Read the model definition and answer for the solid it produces. Units are mm, in the model's axes. A direction names the side the tool comes from. Give positions to 0.01 mm unless a question says otherwise; leave off trailing zeros. Order: outer loops, then holes, each group sorted by start corner. A loop starts at its lowest first (then second) coordinate and runs counter-clockwise, first axis right, second up. Notation, with made-up numbers: M 71.25,-34 L 104.25,-34 A17 cw 104.25,-5 Z; hole C 86.5,-12.75 d4. An arc over 180 degrees is marked long. One line per item, written item: value.
Solid Edge part; units mm, degrees
sketch "Sketch1" plane through (0, 0, 0) normal (0, 0, 1) x (1, 0, 0)
  circle A0 centre (0, 0) radius 62.5
  circle A1 centre (-39.7748, -39.7748) radius 1.5
  circle A2 centre (39.7748, -39.7748) radius 1.5
  circle A3 centre (39.7748, 39.7748) radius 1.5
  circle A4 centre (-39.7748, 39.7748) radius 1.5
extrude "Protrusion1" add sketch "Sketch1" along normal blind 75
sketch "Sketch2" plane through (0, 0, 75) normal (0, 0, 1) x (1, 0, 0)
  arc A0 (-37.0362, 42.3365) -> (37.0362, 42.3365) centre (0, 0) cw
  arc A1 (42.3365, 37.0362) -> (42.3365, -37.0362) centre (0, 0) cw
  arc A2 (37.0362, -42.3365) -> (-37.0362, -42.3365) centre (0, 0) cw
  arc A3 (-42.3365, -37.0362) -> (-42.3365, 37.0362) centre (0, 0) cw
  arc A4 (-37.0362, 42.3365) -> (-42.3365, 37.0362) centre (-39.7748, 39.7748) cw
  arc A5 (42.3365, 37.0362) -> (37.0362, 42.3365) centre (39.7748, 39.7748) cw
  arc A6 (37.0362, -42.3365) -> (42.3365, -37.0362) centre (39.7748, -39.7748) cw
  arc A7 (-42.3365, -37.0362) -> (-37.0362, -42.3365) centre (-39.7748, -39.7748) cw
extrude "ExtrudedCutout_1" cut sketch "Sketch2" against normal blind 30
sketch "Sketch3" plane through (0, -62.5, 37.5) normal (0, -1, 0) x (0, 0, -1)
  line L0 (15, 15) -> (15, -15)
  line L1 (15, -15) -> (35, -15)
  line L2 (35, -15) -> (35, 15)
  line L3 (35, 15) -> (15, 15)
extrude "ExtrudedCutout_2" cut sketch "Sketch3" against normal blind 65
sketch "Sketch4" plane through (0, 0, 45) normal (0, 0, 1) x (1, 0, 0)
  line L0 (-20, -52.5744) -> (-15, -52.5744)
  line L1 (-15, -52.5744) -> (-15, -47.5744)
  line L2 (-15, -47.5744) -> (-20, -47.5744)
  line L3 (-20, -47.5744) -> (-20, -52.5744)
  line L4 (20, -52.5744) -> (15, -52.5744)
  line L5 (15, -52.5744) -> (15, -47.5744)
  line L6 (15, -47.5744) -> (20, -47.5744)
  line L7 (20, -47.5744) -> (20, -52.5744)
extrude "Cutout1" cut sketch "Sketch4" against normal up to vertex (42.5 mm away)
sketch "Sketch5" plane through (0, -62.5, 37.5) normal (0, -1, 0) x (0, 0, -1)
  line L0 (-37.5, 20) -> (37.5, 20)
  line L1 (37.5, 20) -> (37.5, -20)
  line L2 (37.5, -20) -> (-37.5, -20)
  line L3 (-37.5, -20) -> (-37.5, 20)
extrude "Cutout2" cut sketch "Sketch5" against normal up to vertex (9.9256 mm away)
sketch "Sketch6" plane through (0, -52.5744, 33.75) normal (0, -1, 0) x (1, 0, 0)
  circle A0 centre (0, 3.75) radius 1.4
extrude "ExtrudedCutout_5" cut sketch "Sketch6" against normal blind 17.4909
fillet "Round_1" radius 2 1 edges at (-1.4, -52.5744, 37.5)
sketch "Sketch7" plane through (0, 1.6432, 75) normal (0, 0, 1) x (0, 1, 0)
  arc A0 (-38.7663, -37.1231) -> (-50.1844, -20) centre (-1.6432, 0) cw
  line L0 (-54.2176, -20) -> (-50.1844, -20)
  arc A1 (-43.9797, -37.0362) -> (-54.2176, -20) centre (-1.6432, 0) cw
  line L1 (-43.9797, -37.0362) -> (-38.7663, -37.1231)
extrude "Protrusion2" add sketch "Sketch7" against normal up to vertex (30 mm away)
sketch "Sketch8" plane through (31.25, -54.1266, 37.5) normal (0.5, -0.866, 0) x (0, 0, -1)
  line L0 (-10, -5) -> (-35, -5)
  line L1 (-35, -5) -> (-35, 5)
  line L2 (-35, 5) -> (-10, 5)
  line L3 (-10, 5) -> (-10, -5)
extrude "ExtrudedCutout_7" cut sketch "Sketch8" against normal blind 5.5
sketch "Sketch9" plane through (28.5, -49.3634, 60) normal (0.5, -0.866, 0) x (0.866, 0.5, 0)
  line L0 (-5, 5.75) -> (5, 5.75)
  line L1 (5, 5.75) -> (5, -5.75)
  line L2 (5, -5.75) -> (-5, -5.75)
  line L3 (-5, -5.75) -> (-5, 5.75)
  circle A0 centre (0, 7.6) radius 1
  circle A1 centre (0, -7.6) radius 1
extrude "Cutout3" cut sketch "Sketch9" against normal up to next
1) Determine the mould class of faces 1 (the face through (31.66, -44.84, 60.08)), 2 (the face through (20, -55, 30)), 3 (the face through (37.07, 37.18, 60.21)) for opening direction Y: +Y half, -Y half, draft (parallel to the pull), parting line (faces both ways), or undercut.
Reported:
face 1: -Y half
face 2: draft
face 3: undercut
2) Find section B-B, the plane y = 0. Write down the section's boundary in (x, z), plus the area to 3 significant figures.
Reported:
outline: M -62.5,0 L 62.5,0 L 62.5,75 L 56.25,75 L 56.25,45 L -56.25,45 L -56.25,75 L -62.5,75 Z; hole M -15,2.5 L 15,2.5 L 15,22.5 L -15,22.5 Z
area: 5,400 mm^2
3) Each of these flat-tipped pins is pushed along its axis until it touches: pin 1 Ø1 at (y, z) = (38.5, 50) entering from -X; pin 2 Ø5 at (x, z) = (-11.5, 41) entering from -Y; pin 3 Ø3 at (x, z) = (-37, 53.5) entering from -Y. Where does it stop, or does it pass through?
Reported:
pin 1: stops at x = -49.62
pin 2: stops at y = -52.57
pin 3: stops at y = -51.44
4) Which of the six approach directions +Z, -Z, +X, -X, +Y, -Y give full straight-line access (tool end or side, diameter ignored) to faces 4 (the face through (25.513, -54.19, 59.825)), 5 (the face through (27, -47, 54.25)), 6 (the face through (0, 2.5, 13))?
Reported:
face 4: +X
face 5: none
face 6: -Y
5) Find section A-A, the plane z = 62. Count the separate pieces of the cut face and the enclosed holes in it, plus the area to 3 significant figures.
Reported:
separate pieces: 2
enclosed holes: 4
area: 2,110 mm^2
6) Find section D-D, the plane z = 19.5. Write down the section's boundary in (x, y), plus the area to 3 significant figures.
Reported:
outline: M -20,-59.21 L -20,-47.57 L -15,-47.57 L -15,2.5 L 15,2.5 L 15,-47.57 L 20,-47.57 L 20,-59.21 A62.5 ccw long Z; hole C -39.77,-39.77 d3; hole C -39.77,39.77 d3; hole C 39.77,-39.77 d3; hole C 39.77,39.77 d3
area: 10,200 mm^2
7) Find section C-C, the plane x = -9. Write down the section's boundary in (y, z).
Reported:
outline: M -52.57,0 L 61.85,0 L 61.85,75 L 55.53,75 L 55.53,45 L -52.57,45 L -52.57,22.5 L 2.5,22.5 L 2.5,2.5 L -52.57,2.5 Z
8) Consider probe 1 along Z at (x, y) = (0, -47); probe 2 along Z at (x, y) = (7, -40); probe 3 along X at (y, z) = (36.5, 72.5). Determine where each line is inside the solid, lowest interval first.
Reported:
probe 1: z = 0 to 2.5, 22.5 to 36.1, 38.9 to 45
probe 2: z = 0 to 2.5, 22.5 to 45
probe 3: x = -50.73 to -42.8, -41.6 to -37.95, 37.95 to 41.6, 42.8 to 50.73
